from build123d import *

# Parameters (mm, degrees)
F0_W      = 30
F0_H      = 12
F0_R      = 1.5
F1_DEPTH  = 33
F2_W      = 12
F2_H      = 28
F3_DEPTH  = 25
F4_R      = 2.65
F5_DEPTH  = 28.5
F6_R      = 5
F7_R      = 1
F8_R      = 2.05
F8_R_2    = 1.5
F9_DEPTH  = 25
F10_SIZE2 = 7.5
F10_SIZE  = 3
F11_W     = 6
F11_H     = 28
F12_DEPTH = 25
F13_R     = 2


with BuildPart() as f1:
    # F0 (on Top) → F1 (new body)
    with BuildSketch(Plane.XY):
        with Locations((15, 6)):
            Rectangle(F0_W, F0_H)
        with Locations((24, 6)):
            Circle(F0_R, mode=Mode.SUBTRACT)
    extrude(amount=F1_DEPTH)

    # F2 (on face) → F3 (cut)
    with BuildSketch(Plane.XZ):
        with Locations((6, 16.5)):
            Rectangle(F2_W, F2_H)
    extrude(amount=-F3_DEPTH, mode=Mode.SUBTRACT)

    # F4 (on face) → F5 (join)
    with BuildSketch(Plane.XY.offset(2.5)):
        with Locations((6, 6)):
            Circle(F4_R)
    extrude(amount=F5_DEPTH)

    # F6
    f6_edges = [f1.edges().sort_by_distance(p)[0] for p in [
        (0, 0, 1.25),
        (0, 0, 31.75),
        (0, 12, 1.25),
        (0, 12, 31.75),
        (30, 0, 16.5),
        (30, 12, 16.5),
    ]]
    fillet(f6_edges, radius=F6_R)

    # F7
    f7_edges = [f1.edges().sort_by_distance(p)[0] for p in [
        (12, 6, 2.5),
        (12, 6, 30.5),
    ]]
    fillet(f7_edges, radius=F7_R)

    # F8 (on face) → F9 (cut)
    with BuildSketch(Plane.XY.offset(33)):
        with Locations((24, 6)):
            Circle(F8_R)
        with Locations((24, 6)):
            Circle(F8_R_2, mode=Mode.SUBTRACT)
    extrude(amount=-F9_DEPTH, mode=Mode.SUBTRACT)

    # F10
    f10_edges = [f1.edges().sort_by_distance(p)[0] for p in [
        (22.5, 6, 0),
    ]]
    chamfer(f10_edges, length=F10_SIZE, length2=F10_SIZE2)

    # F11 (on face) → F12 (cut)
    with BuildSketch(Plane.XZ):
        with Locations((17, 16.5)):
            Rectangle(F11_W, F11_H)
    extrude(amount=-F12_DEPTH, mode=Mode.SUBTRACT)

    # F13
    f13_edges = [f1.edges().sort_by_distance(p)[0] for p in [
        (14, 6, 30.5),
        (20, 6, 30.5),
        (14, 6, 2.5),
        (20, 6, 2.5),
    ]]
    fillet(f13_edges, radius=F13_R)


solid = f1.part
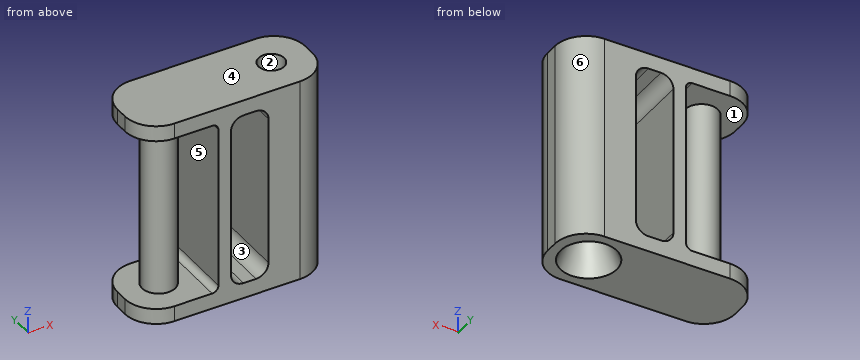
Model file for the job. Use its own axes, mm. Face numbers are marked on the shaded views. A direction names the side the tool comes from. Give positions to 0.01 mm unless a question says otherwise; leave off trailing zeros. Order: outer loops, then holes, each group sorted by start corner. A loop starts at its lowest first (then second) coordinate and runs counter-clockwise, first axis right, second up. Notation, with made-up numbers: M 24.25,36 L 42.25,36 A9 ccw 42.25,40 Z; hole C -34,48.25 d8. An arc over 180 degrees is marked long. Write item = value, one per line.
Q1. Drill centre lines: line 1 (Z direction, x = 3.5, y = 3.5); line 2 (Y direction, x = 24, z = 7.65); line 3 (Y direction, x = 24, z = 26.25). Where is each one in solid material? Low to high. Write a range as [from, to].
Derived:
line_1 = [0, 2.5], [30.5, 33]
line_2 = [0, 4.5], [7.5, 12]
line_3 = [0, 3.95], [8.05, 12]
Q2. Flat gauge pins, fed straight in: pin 1 (3.5 mm diameter, centred on y = 5, z = 12.5, fed in from -X); pin 2 (3.5 mm diameter, centred on x = 24, y = 6, fed in from +Z); pin 3 (1.5 mm diameter, centred on x = 10.5, z = 10, fed in from -Y); pin 4 (1 mm diameter, centred on y = 10, z = 17, fed in from -X). Where does each tip first touch, or does it go through?
Derived:
pin_1 = 3.35
pin_2 = 8
pin_3 = through
pin_4 = 12
Q3. Two-plate mould, pull along Z, no slides. Class the marked faces 4, 5 and 6: pulls with the +Z half, pulls with the -Z half, needs draft (parallel to the pull), parting line crosses it, or undercut.
Derived:
face_4 = pulls with the +Z half
face_5 = undercut
face_6 = needs draft
Q4. Cut at D-D, the plane x = 6. List the corners of the cut face in (y, z).
Derived:
outline = M 0,0 L 12,0 L 12,2.5 L 8.65,2.5 L 8.65,30.5 L 12,30.5 L 12,33 L 0,33 L 0,30.5 L 3.35,30.5 L 3.35,2.5 L 0,2.5 Z
Q5. Cut at C-C, the plane x = 10. List the corners of the cut face in (y, z).
Derived:
outline = M 0,0 L 12,0 L 12,2.5 L 0,2.5 Z; M 0,30.5 L 12,30.5 L 12,33 L 0,33 Z
Q6. Tool access for the marked faces 1, 2 and 3: list every direction of +Z, -Z, +X, -X, +Y, -Y with a clear straight run to the whole face (end or side of a thin tool).
Derived:
face_1 = none
face_2 = +Z
face_3 = +Y, -Y
Q7. Cut at B-B, the plane z = 24.5. List the corners of the cut face in (x, y), then the cut area to 3 significant figures.
Derived:
outline = C 6,6 d5.3; M 12,0 L 14,0 L 14,12 L 12,12 Z; M 20,0 L 25,0 A5 ccw 30,5 L 30,7 A5 ccw 25,12 L 20,12 Z; hole C 24,6 d4.1
area = 142 mm2
Q8. Cut at A-A, the plane y = 6. Count the separate pieces of the cut face and the enclosed holes in it, then the cut area to 3 significant figures.
Derived:
separate_pieces = 2
enclosed_holes = 2
area = 489 mm2
